CAD build for the part. Positions are in the model's coordinates, mm. Face numbers are marked on the shaded views. A direction names the side the tool comes from. Coordinates: 2 decimals unless noted, no trailing zeros. Order: outer loops, then holes, each group sorted by start corner. A loop starts at its lowest first (then second) coordinate and runs counter-clockwise, first axis right, second up. Notation, with made-up numbers: M -28,-8 L -22,-8 A28 cw -22,21 Z; hole C 23,24 d2. An arc over 180 degrees is marked long. One line per item, written item: value.
from build123d import *

# Parameters (mm, degrees)
F1_DEPTH = 53.975
F3_DEPTH = 101.6


with BuildPart() as f1:
    # F0 (on Top) → F1 (new body)
    with BuildSketch(Plane.XY):
        Polygon((36.5125, -50.8), (76.2, -50.8), (76.2, 50.8), (-76.2, 50.8), (-76.2, 25.4), (25.4, 25.4), (25.4, 36.5125), (47.625, 36.5125), (47.625, 14.2875), (36.5125, 14.2875), align=None)
        with BuildLine():
            Line((-76.2, -50.8), (0, -50.8))
            Line((0, -50.8), (0, -12.7))
            ThreePointArc((0, -12.7), (-8.9802561211, -8.9802561211), (-12.7, 0))
            Line((-12.7, 0), (-76.2, 0))
            Line((-76.2, 0), (-76.2, -12.7))
            Line((-76.2, -12.7), (-50.8, -12.7))
            ThreePointArc((-50.8, -12.7), (-41.8197438789, -16.4197438789), (-38.1, -25.4))
            ThreePointArc((-38.1, -25.4), (-41.8197438789, -34.3802561211), (-50.8, -38.1))
            Line((-50.8, -38.1), (-76.2, -38.1))
            Line((-76.2, -38.1), (-76.2, -50.8))
        make_face()
        with BuildLine():
            Line((0, -50.8), (36.5125, -50.8))
            Line((36.5125, -50.8), (36.5125, 14.2875))
            Line((36.5125, 14.2875), (25.4, 14.2875))
            Line((25.4, 14.2875), (25.4, 25.4))
            Line((25.4, 25.4), (-76.2, 25.4))
            Line((-76.2, 25.4), (-76.2, 0))
            Line((-76.2, 0), (-12.7, 0))
            ThreePointArc((-12.7, 0), (0, 12.7), (12.7, 0))
            ThreePointArc((12.7, 0), (8.9802561211, -8.9802561211), (0, -12.7))
            Line((0, -12.7), (0, -50.8))
        make_face()
    extrude(amount=F1_DEPTH)

    # F2 (on face) → F3 (cut)
    with BuildSketch(Plane.XZ.offset(50.8)):
        Polygon((-76.2, 23.8125), (76.2, 53.975), (-76.2, 53.975), align=None)
    extrude(amount=-F3_DEPTH, mode=Mode.SUBTRACT)


solid = f1.part
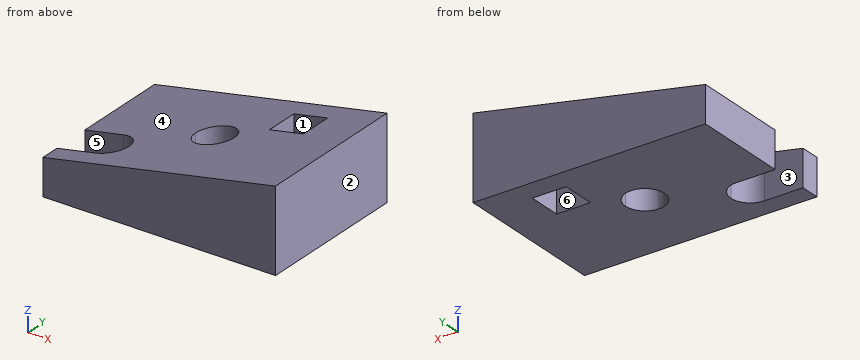
Q1. Slice it at B-B (y = 3). List the corners of the cut face in (x, z) (1 decimal), plus the area to 3 significant figures.
Recorded:
outline: M -76.2,0 L -12.3,0 L -12.3,36.5 L -76.2,23.8 Z; M 12.3,0 L 76.2,0 L 76.2,54 L 12.3,41.3 Z
area: 4,970 mm^2
Q2. Mould opens along X. For the marked faces 1, 2 and 3 say: released by +X, released by -X, zero draft, split by the parting line, or undercut.
Recorded:
face 1: undercut
face 2: released by +X
face 3: zero draft
Q3. Slice it at D-D (z = 50). List the corners of the cut face in (x, y), plus the area to 3 significant figures.
Recorded:
outline: M 56.12,-50.8 L 76.2,-50.8 L 76.2,50.8 L 56.12,50.8 Z
area: 2,040 mm^2
Q4. Which spindle directions (+Z, -Z, +X, -X, +Y, -Y) get a long thin tool onto all of the face, cutting with end or side? Do the marked faces 4, 5 and 6. Say none if no direction does.
Recorded:
face 4: +Z, -X, +Y, -Y
face 5: +Z, -Z, -X
face 6: +Z, -Z
Q5. Slice it at C-C (x = -6.5). List the corners of the cut face in (y, z).
Recorded:
outline: M -50.8,0 L -10.91,0 L -10.91,37.61 L -50.8,37.61 Z; M 10.91,0 L 50.8,0 L 50.8,37.61 L 10.91,37.61 Z
Q6. Slice it at A-A (z = 14.5). List the corners of the cut face in (x, y) (1 decimal).
Recorded:
outline: M -76.2,-50.8 L 76.2,-50.8 L 76.2,50.8 L -76.2,50.8 L -76.2,-12.7 L -50.8,-12.7 A12.7 cw -50.8,-38.1 L -76.2,-38.1 Z; hole C 0,0 d25.4; hole M 25.4,14.3 L 47.6,14.3 L 47.6,36.5 L 25.4,36.5 Z
Q7. Drill centre lines: line 1 along X through (y, z) = (19, 15) (3 decimals); line 2 along Y through (x, z) = (-55, 16.5); line 3 along Z through (x, y) = (-12, 36.5). Where is each one in solid material? Low to high.
Recorded:
line 1: x = -76.2 to 25.4, 47.625 to 76.2
line 2: y = -50.8 to -38.1, -12.7 to 50.8
line 3: z = 0 to 36.52
